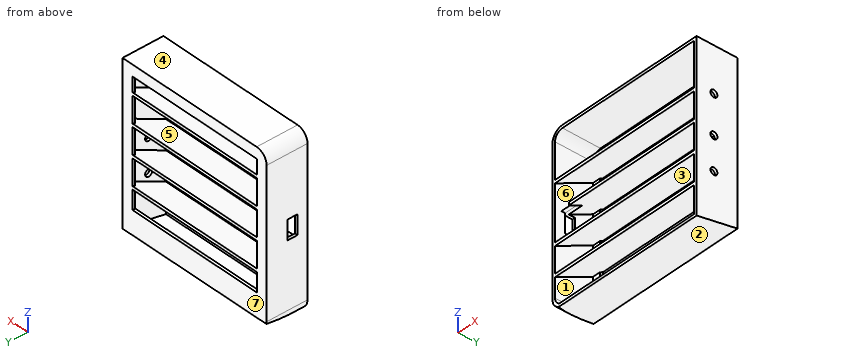
from build123d import *

# Parameters (mm, degrees)
F1_DEPTH    = 37
F2_T1_DEPTH = 342.8505669038
F3_T        = -2.54
F4_W        = 125.55387271
F4_H        = 111.9176980871
F5_DEPTH    = 25.4
F6_R        = 3.175
F7_DEPTH    = 19.05
F9_DEPTH    = 142.24
F10_W       = 9
F10_H       = 17.5
F11_DEPTH   = 16.5
F13_DEPTH   = 14


# Not quite as in the source:
# - a fillet or chamfer that OpenCascade refuses, or shapes differently, is made with other operations: its cross-section is extruded or revolved along the edge and cut away or added
# - a feature names something its author has since deleted; it is built from what else it names


with BuildPart() as f1:
    # F0 (on Front) → F1 (new body)
    with BuildSketch(Plane.XZ):
        with BuildLine():
            Line((72.5, 75.5), (-62.5, 75.5))
            ThreePointArc((-62.5, 75.5), (-69.5710678119, 72.5710678119), (-72.5, 65.5))
            Line((-72.5, 65.5), (-72.5, -65.5))
            ThreePointArc((-72.5, -65.5), (-69.5710678119, -72.5710678119), (-62.5, -75.5))
            Line((-62.5, -75.5), (72.5, -75.5))
            Line((72.5, -75.5), (72.5, 75.5))
        make_face()
    extrude(amount=F1_DEPTH)

    # F2: chamfer of 40 x 8 on 1 edges, made by hand

    # F2_s2 → F2_t1 (cut)
    with BuildSketch(Plane.YZ.offset(-166.4252834519)):
        Polygon((-40, -75.5), (0, -67.5), (0, -75.5), align=None)
    extrude(amount=F2_T1_DEPTH, mode=Mode.SUBTRACT)

    # F3
    f3_openings = [f1.faces().sort_by_distance(p)[0] for p in [
        (0.123954, -37, 0.284541),
    ]]
    offset(amount=F3_T, openings=f3_openings)

    # F4 (on face) → F5 (cut)
    with BuildSketch(Plane.XZ.offset(2.54)):
        with Locations((-0.276936355, 9.5411509565)):
            Rectangle(F4_W, F4_H)
    extrude(amount=-F5_DEPTH, mode=Mode.SUBTRACT)

    # F6 (on face) → F7 (cut)
    with BuildSketch(Plane(origin=(69.96, 0, 0), x_dir=(0, -1, 0), z_dir=(-1, 0, 0))):
        with Locations((21.3561020792, 0)):
            Circle(F6_R)
        with Locations((21.3561020792, 35)):
            Circle(F6_R)
        with Locations((21.3561020792, -30)):
            Circle(F6_R)
    extrude(amount=-F7_DEPTH, mode=Mode.SUBTRACT)

    # F8 (on face) → F9 (join)
    with BuildSketch(Plane(origin=(69.96, 0, 0), x_dir=(0, -1, 0), z_dir=(-1, 0, 0))):
        Polygon((0, -29.2355429628), (37, -47.9510980871), (37, -45.1046433113), (0, -26.389088187), align=None)
        Polygon((0, -3.021088187), (37, -21.7366433113), (37, -18.8901885355), (0, -0.1746334112), align=None)
        Polygon((0, 23.1933665888), (37, 4.4778114645), (37, 7.3242662403), (0, 26.0398213646), align=None)
        Polygon((0, 49.4078213646), (37, 30.6922662403), (37, 33.5387210161), (0, 52.2542761405), align=None)
    extrude(amount=F9_DEPTH)

    # F10 (on face) → F11 (cut)
    with BuildSketch(Plane(origin=(-72.5, 0, 0), x_dir=(0, -1, 0), z_dir=(-1, 0, 0))):
        with Locations((23.4, 2)):
            Rectangle(F10_W, F10_H)
    extrude(amount=-F11_DEPTH, mode=Mode.SUBTRACT)

    # F12 (on face) → F13 (cut)
    with BuildSketch(Plane.YZ.offset(-69.96)):
        Polygon((-44.6556091905, -6.75), (-37, -6.75), (-37, 4.4778114645), (-27.9, 9.0808263735), (-27.9, 10.2238561958), (-44.6556091905, 10.2238561958), align=None)
    extrude(amount=F13_DEPTH, mode=Mode.SUBTRACT)


solid = f1.part
Work out the finished part from the listing and answer in its coordinate system (mm). Face numbers are marked on the shaded views. A direction names the side the tool comes from. Give positions to 0.01 mm unless a question says otherwise; leave off trailing zeros. Order: outer loops, then holes, each group sorted by start corner. A loop starts at its lowest first (then second) coordinate and runs counter-clockwise, first axis right, second up. Notation, with made-up numbers: (-36, 50) - (-7, 50) arc R35 cw to (-7, 88) - close; hole circle Ø7 at (67, 42). An arc over 180 degrees is marked (long way). Answer as CSV lines item,"result". Start each with the question number.
Q1. The part is cut by section C-C (y = -21). Give the number of separate pieces and of enclosed holes in the cut face, then the cut area to 3 significant figures.
Q2. The mould has two halves that part along Z. Classify the marked faces 1, 2, 3 and 4: +Z half, -Z half, draft (parallel to the pull), parting line (faces both ways), or undercut.
Q3. The part is cut by section A-A (x = 37.5). Write down the section's boundary in (y, z), then the cut area to 3 significant figures.
Q4. The part is cut by section B-B (z = -59.5). Write down the section's boundary in (x, y).
Q5. For the marked faces 5, 6 and 7, determine the directions among +Z, -Z, +X, -X, +Y, -Y from which every point of the face is accessible in a straight line to the end or side of a thin tool.
Q6. Find the intervals of material crossed by L1, parallel to X at y = -30, z = -53; L2, parallel to Z at x = 38.5, y = -18.5; L3, parallel to Z at x = 35, y = -14, in increasing order. Write a range as [from, to].
Q7. Given pin 1 Ø6 at (x, z) = (66, -15.5) entering from -Y; pin 2 Ø1 at (x, y) = (46.5, -6) entering from -Z; pin 3 Ø1 at (x, z) = (-3, -8) entering from -Y, each flat-ended and moving along its own axis, determine where each tip first touches the part or whether it passes through.
Check result:
1,separate pieces,"2"
1,enclosed holes,"2"
1,area,"2,950 mm²"
2,face 1,"undercut"
2,face 2,"-Z half"
2,face 3,"undercut"
2,face 4,"+Z half"
3,outline,"(-37, -74.9) - (0, -67.5) - (0, -46.42) - (-2.54, -46.42) - (-2.54, -65.42) - (-37, -72.31) - close; (-37, -47.95) - (0, -29.24) - (0, -26.39) - (-37, -45.1) - close; (-37, -21.74) - (0, -3.02) - (0, -0.17) - (-37, -18.89) - close; (-37, 4.48) - (0, 23.19) - (0, 26.04) - (-37, 7.32) - close; (-37, 30.69) - (0, 49.41) - (0, 52.25) - (-37, 33.54) - close; (-37, 72.96) - (-2.54, 72.96) - (-2.54, 65.5) - (0, 65.5) - (0, 75.5) - (-37, 75.5) - close"
3,area,"678 mm²"
4,outline,"(-72.5, -37) - (-69.96, -37) - (-69.96, -2.54) - (69.96, -2.54) - (69.96, -37) - (72.5, -37) - (72.5, 0) - (-72.5, 0) - close"
5,face 5,"-Y"
5,face 6,"none"
5,face 7,"+Z, -Z, +X, -X, +Y"
6,L1,"x = [-72.5, -69.96], [69.96, 72.5]"
6,L2,"z = [-71.2, -68.61], [-38.59, -35.75], [-12.38, -9.53], [13.84, 16.68], [40.05, 42.9], [72.96, 75.5]"
6,L3,"z = [-70.3, -67.71], [-36.32, -33.47], [-10.1, -7.26], [16.11, 18.96], [42.33, 45.17], [72.96, 75.5]"
7,pin 1,"stops at y = -36.23"
7,pin 2,"stops at z = -68.8"
7,pin 3,"stops at y = -16.46"
